Autodesk Inventor part; units mm, degrees
ref_plane "YZ Plane" through (0, 0, 0) normal (1, 0, 0) x (0, 1, 0)
ref_plane "XZ Plane" through (0, 0, 0) normal (0, 1, 0) x (-1, 0, 0)
ref_plane "XY Plane" through (0, 0, 0) normal (0, 0, 1) x (1, 0, 0)
sketch "Esboço1" plane through (0, 0, 0) normal (0, 0, 1) x (1, 0, 0)
  line L0 (0, 0) -> (20, 0)
  line L1 (20, 0) -> (20, 20)
  line L2 (20, 20) -> (0, 20)
  line L3 (0, 20) -> (0, 0)
  dimension "d0" = 20
  dimension "d1" = 20
extrude "Extrusão1" add sketch "Esboço1" along normal blind 1
sketch "Esboço2" plane through (0, 0, 1) normal (0, 0, 1) x (1, 0, 0)
  line L0 (0.9, 15) -> (1.4, 15)
  line L1 (1.4, 15) -> (1.4, 13.5)
  line L2 (1.4, 13.5) -> (0.9, 13.5)
  line L3 (0.9, 13.5) -> (0.9, 15)
  line L4 (0.9, 5) -> (1.4, 5)
  line L5 (1.4, 5) -> (1.4, 6.5)
  line L6 (1.4, 6.5) -> (0.9, 6.5)
  line L7 (0.9, 6.5) -> (0.9, 5)
  line L8 (0, 20) -> (0, 0)
  line L9 (0, 0) -> (20, 0)
  line L10 (20, 20) -> (0, 20)
  line L11 (10, 20) -> (10, 0)
  line L12 (19.1, 15) -> (18.6, 15)
  line L13 (18.6, 15) -> (18.6, 13.5)
  line L14 (18.6, 13.5) -> (19.1, 13.5)
  line L15 (19.1, 13.5) -> (19.1, 15)
  line L16 (19.1, 5) -> (18.6, 5)
  line L17 (18.6, 5) -> (18.6, 6.5)
  line L18 (18.6, 6.5) -> (19.1, 6.5)
  line L19 (19.1, 6.5) -> (19.1, 5)
  dimension "d4" = 1.5
  dimension "d5" = 0.5
  dimension "d6" = 0.5
  dimension "d7" = 1.5
  dimension "d8" = 0.9
  dimension "d9" = 5
  dimension "d10" = 5
extrude "Extrusão2" add sketch "Esboço2" along normal blind 1 contours L0 L1 L2 L3 | L7 L6 L5 L4 | L15 L14 L13 L12 | L16 L17 L18 L19
sketch "Esboço3" plane through (0, 0, 1) normal (0, 0, 1) x (1, 0, 0)
  line L0 (0, 0) -> (20, 0)
  line L1 (8, 0) -> (12, 0)
  line L2 (12, 0) -> (12, -3)
  line L3 (12, -3) -> (8, -3)
  line L4 (8, -3) -> (8, 0)
  dimension "d13" = 8
  dimension "d14" = 8
  dimension "d15" = 3
extrude "Extrusão3" add sketch "Esboço3" against normal blind 1
properties part number "caixaled_pt2" material "Plástico PC/ABS"
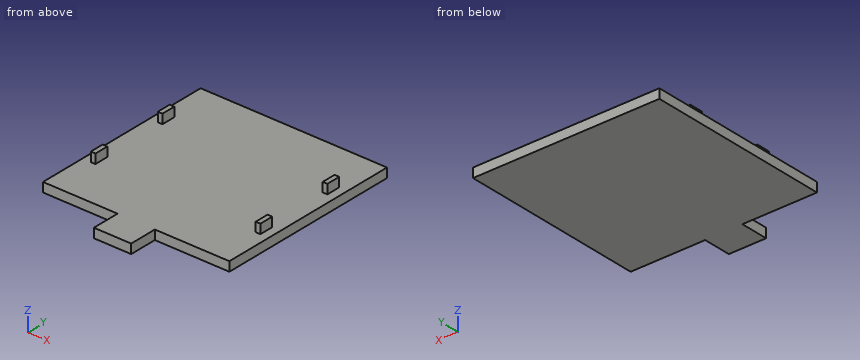
CAD build for the part. Positions are in the model's coordinates, mm. Give positions to 0.01 mm unless a question says otherwise; leave off trailing zeros. Order: outer loops, then holes, each group sorted by start corner. A loop starts at its lowest first (then second) coordinate and runs counter-clockwise, first axis right, second up.
(1) Saw through at A-A, the plane z = 0.65. Give the cut face in (x, y).
(2) Flat gauge pins, fed straight in: pin 1 (0.5 mm diameter, centred on y = 14, z = 1.5, fed in from -X); pin 2 (0.5 mm diameter, centred on x = 14, z = 0.5, fed in from -Y); pin 3 (3 mm diameter, centred on x = 6, y = 16.5, fed in from +Z). Where does each tip first touch, or does it go through?
(3) Saw through at C-C, the plane x = 8.5. Give the cut face in (y, z).
(4) Drill centre lines: L1, parallel to Z at x = 2.25, y = 1.5; L2, parallel to Y at x = 4, z = 0.7. Where is each one in solid material? Low to high.
(5) Saw through at B-B, the plane y = 3. Give the cut face in (x, z), then the cut area to 3 significant figures.
Results found:
1. outline: (0, 0) - (8, 0) - (8, -3) - (12, -3) - (12, 0) - (20, 0) - (20, 20) - (0, 20) - close
2. pin 1: stops at x = 0.9
2. pin 2: stops at y = 0
2. pin 3: stops at z = 1
3. outline: (-3, 0) - (20, 0) - (20, 1) - (-3, 1) - close
4. L1: z = 0 to 1
4. L2: y = 0 to 20
5. outline: (0, 0) - (20, 0) - (20, 1) - (0, 1) - close
5. area: 20.0 mm2
